Geometry check sheet. Reference: the model listing, model coordinates, mm. Give positions to 0.01 mm unless a question says otherwise; leave off trailing zeros. Order: outer loops, then holes, each group sorted by start corner. A loop starts at its lowest first (then second) coordinate and runs counter-clockwise, first axis right, second up. Notation, with made-up numbers: (35, -25.75) - (90, -25.75) arc R27 cw to (90, 10.25) - close; hole circle Ø11 at (-24, -12.75). An arc over 180 degrees is marked (long way). Put each result on its own line as item: value. Start each with the question number.
```python
from build123d import *

# Parameters (mm, degrees)
CENTERSKETCH1_W            = 210
CENTERSKETCH1_H            = 210
CENTERBOSS_EXTRUDE1_DEPTH  = 20
TABHOLESSKETCH1_R          = 1
TABHOLESCUT_EXTRUDE1_DEPTH = 17
CHAMFER1_SIZE              = 20


with BuildPart() as part:
    # CenterSketch1 → CenterBoss-Extrude1 (new body)
    with BuildSketch(Plane(origin=(0, 0, 0), x_dir=(1, 0, 0), z_dir=(0, 1, 0))):
        with Locations((105, 105)):
            Rectangle(CENTERSKETCH1_W, CENTERSKETCH1_H)
    extrude(amount=CENTERBOSS_EXTRUDE1_DEPTH)

    # TabHolesSketch1 → TabHolesCut-Extrude1 (cut)
    with BuildSketch(Plane(origin=(0, 20, 0), x_dir=(1, 0, 0), z_dir=(0, 1, 0))):
        with Locations(Location((10, 10, 0), (0, 0, 270))):
            Circle(TABHOLESSKETCH1_R)
        with Locations(Location((200, 10, 0), (0, 0, 270))):
            Circle(TABHOLESSKETCH1_R)
        with Locations(Location((200, 200, 0), (0, 0, 270))):
            Circle(TABHOLESSKETCH1_R)
        with Locations(Location((10, 200, 0), (0, 0, 270))):
            Circle(TABHOLESSKETCH1_R)
        with Locations(Location((65, 200, 0), (0, 0, 270))):
            Circle(TABHOLESSKETCH1_R)
        with Locations(Location((120, 200, 0), (0, 0, 270))):
            Circle(TABHOLESSKETCH1_R)
        with Locations(Location((160, 200, 0), (0, 0, 270))):
            Circle(TABHOLESSKETCH1_R)
        with Locations(Location((10, 160, 0), (0, 0, 270))):
            Circle(TABHOLESSKETCH1_R)
        with Locations(Location((10, 65, 0), (0, 0, 270))):
            Circle(TABHOLESSKETCH1_R)
        with Locations(Location((10, 120, 0), (0, 0, 270))):
            Circle(TABHOLESSKETCH1_R)
        with Locations(Location((50, 10, 0), (0, 0, 270))):
            Circle(TABHOLESSKETCH1_R)
        with Locations(Location((90, 10, 0), (0, 0, 270))):
            Circle(TABHOLESSKETCH1_R)
        with Locations(Location((145, 10, 0), (0, 0, 270))):
            Circle(TABHOLESSKETCH1_R)
        with Locations(Location((200, 145, 0), (0, 0, 270))):
            Circle(TABHOLESSKETCH1_R)
        with Locations(Location((200, 90, 0), (0, 0, 270))):
            Circle(TABHOLESSKETCH1_R)
        with Locations(Location((200, 50, 0), (0, 0, 270))):
            Circle(TABHOLESSKETCH1_R)
    extrude(amount=-TABHOLESCUT_EXTRUDE1_DEPTH, mode=Mode.SUBTRACT)

    # Chamfer1
    # the kernel refuses this chamfer: 20 mm, written as the material it takes off along each edge
    with BuildSketch(Plane(origin=(-51.433659759, 20, 0), x_dir=(0, -0.9996219169112968, 0.027495876610586372), z_dir=(1, 0, 0)), Plane(origin=(210, 20, 51.433659759), x_dir=(0.027495876610586317, -0.9996219169112968, 0), z_dir=(0, 0, -1)), Plane(origin=(0, 20, -261.433659759), x_dir=(-0.027495876610586372, -0.9996219169112968, 0), z_dir=(0, 0, 1))) as chamfer1_piece_1:
        Polygon((CHAMFER1_SIZE * 0.999621916911, CHAMFER1_SIZE * 0.0274958766106), (-CHAMFER1_SIZE * 0.0274958766106, CHAMFER1_SIZE * 0.999621916911), (0, 0), align=None)
    extrude(amount=312.867319519, mode=Mode.SUBTRACT)
    with BuildSketch(Plane(origin=(261.433659759, 20, -210), x_dir=(0, 0.027495876610586317, 0.9996219169112968), z_dir=(-1, 0, 0))) as chamfer1_piece_2:
        Polygon((CHAMFER1_SIZE * 0.999621916911, -CHAMFER1_SIZE * 0.0274958766106), (-CHAMFER1_SIZE * 0.0274958766106, -CHAMFER1_SIZE * 0.999621916911), (0, 0), align=None)
    extrude(amount=312.867319519, mode=Mode.SUBTRACT)


solid = part.part
```
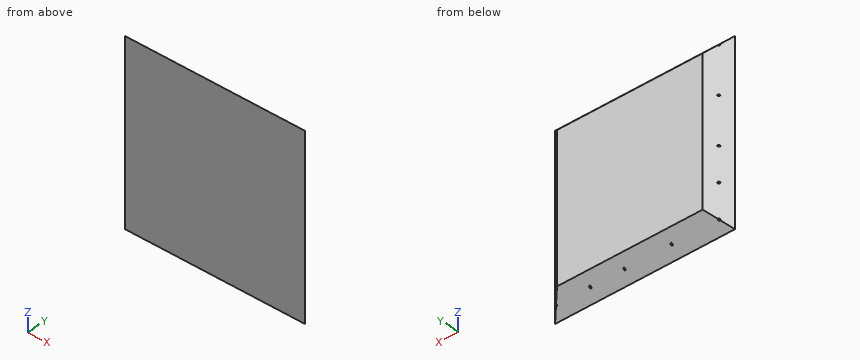
Item 1: Cross-section at A-A (y = 14.75). Enter the section's corners in (x, z), and give its area (3 significant figures).
Item 2: Thickness scan on line 1 along X through (y, z) = (9.25, -10); line 2 along X through (y, z) = (9.5, -200); line 3 along Z through (x, y) = (200, 9.5). Record the ranges inside material, lowest first.
Item 3: Cross-section at B-B (z = -134.5). Enter the section's corners in (x, y), and give its area (3 significant figures).
Item 4: Gauge pin test, flat ends, axial feed: pin 1 Ø2 at (x, z) = (145, -10.5) entering from +Y; pin 2 Ø1.6 at (x, z) = (200, -50) entering from +Y; pin 3 Ø2 at (x, z) = (200, -90.5) entering from +Y. Record the tip position at first contact, or that the pin passes through.
Recorded:
1. outline: (14.75, -195.25) - (195.25, -195.25) - (195.25, -14.75) - (14.75, -14.75) - close
1. area: 32,600 mm^2
2. line 1: x = 11 to 49, 51 to 89, 91 to 144, 146 to 199
2. line 2: x = 11 to 64, 66 to 119, 121 to 159, 161 to 199
2. line 3: z = -199 to -146, -144 to -91, -89 to -51, -49 to -11
3. outline: (0, 0) - (210, 0) - (190, 20) - (20, 20) - close
3. area: 3,800 mm^2
4. pin 1: stops at y = 11.5
4. pin 2: stops at y = 3
4. pin 3: stops at y = 11
